Part model, mm, in its own coordinate system. Coordinates: 2 decimals unless noted, no trailing zeros. Loops run counter-clockwise (first coordinate to the right, second up) from the corner with the lowest first, then second, coordinate; pieces in that order, holes last.
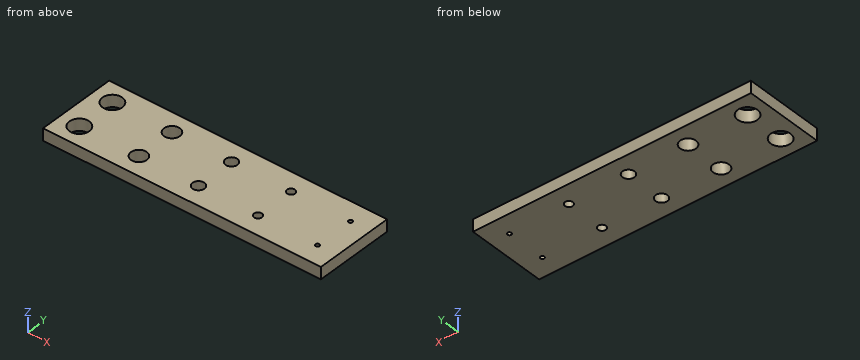
```python
from build123d import *

# Parameters (mm, degrees)
SKETCH_W      = 70
SKETCH_H      = 20
PAD_DEPTH     = 3
SKETCH001_R   = 2.5
SKETCH001_R_2 = 2
SKETCH001_R_3 = 1.5
SKETCH001_R_4 = 1
SKETCH001_R_5 = 0.5
POCKET_DEPTH  = 148.72677


with BuildPart() as part:
    # Sketch → Pad (new body)
    with BuildSketch(Plane.XY):
        Rectangle(SKETCH_W, SKETCH_H)
    extrude(amount=PAD_DEPTH)

    # Sketch001 (on Face6 of Pad) → Pocket (cut, through all)
    with BuildSketch(Plane.XY.offset(3)):
        with Locations((-30, 5)):
            Circle(SKETCH001_R)
        with Locations((-15, 5)):
            Circle(SKETCH001_R_2)
        with Locations((0, 5)):
            Circle(SKETCH001_R_3)
        with Locations((15, 5)):
            Circle(SKETCH001_R_4)
        with Locations((30, 5)):
            Circle(SKETCH001_R_5)
    pocket = extrude(amount=-POCKET_DEPTH, mode=Mode.SUBTRACT)

    # Mirrored: Pocket across XZ
    add(pocket.mirror(Plane.XZ), mode=Mode.SUBTRACT)


solid = part.part
```
Q1. Saw through at C-C (x = 0). List the corners of the cut face in (y, z).
Q2. Saw through at B-B (x = 15). List the corners of the cut face in (y, z), plus the area to 3 significant figures.
Q3. Saw through at A-A (z = 1.55). Count the separate pieces of the cut face and the enclosed holes in it, plus the area to 3 significant figures.
Q4. Drop a flat-ended pin along its axis: P1, Ø8, axis at x = -30, y = -5, coming from the +Z side. Give the stop position or say it passes through.
Q5. Probe line 1 (X direction, y = -5, z = 1.8); line 2 (Y direction, x = 0, z = 1.05); line 3 (X direction, y = 4.75, z = 0.9). List the from-to ranges inside material, lowest first.
Checked values:
1. outline: (-10, 0) - (-6.5, 0) - (-6.5, 3) - (-10, 3) - close; (-3.5, 0) - (3.5, 0) - (3.5, 3) - (-3.5, 3) - close; (6.5, 0) - (10, 0) - (10, 3) - (6.5, 3) - close
2. outline: (-10, 0) - (-6, 0) - (-6, 3) - (-10, 3) - close; (-4, 0) - (4, 0) - (4, 3) - (-4, 3) - close; (6, 0) - (10, 0) - (10, 3) - (6, 3) - close
2. area: 48.0 mm2
3. separate pieces: 1
3. enclosed holes: 10
3. area: 1,310 mm2
4. P1: stops at z = 3
5. line 1: x = -35 to -32.5, -27.5 to -17, -13 to -1.5, 1.5 to 14, 16 to 29.5, 30.5 to 35
5. line 2: y = -10 to -6.5, -3.5 to 3.5, 6.5 to 10
5. line 3: x = -35 to -32.49, -27.51 to -16.98, -13.02 to -1.48, 1.48 to 14.03, 15.97 to 29.57, 30.43 to 35
